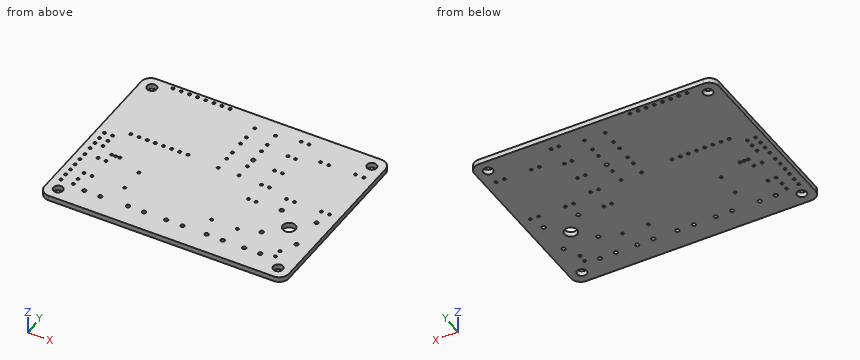
from build123d import *

# Parameters (mm, degrees)
ESQUISSE1_R        = 1.5
ESQUISSE1_R_2      = 0.449122519
ESQUISSE1_R_3      = 0.425258014
ESQUISSE1_R_4      = 0.43212249
ESQUISSE1_R_5      = 0.6
ESQUISSE1_R_6      = 2
BOSS_EXTRU_1_DEPTH = 1.6


with BuildPart() as part:
    # Esquisse1 → Boss.-Extru.1 (new body)
    with BuildSketch(Plane.XY):
        with BuildLine():
            Line((5.620364973, 58.899605158), (75.820364973, 58.899605158))
            ThreePointArc((75.820364973, 58.899605158), (77.941685316, 58.020925502), (78.820364973, 55.899605158))
            Line((78.820364973, 55.899605158), (78.820364973, 3.479605158))
            ThreePointArc((78.820364973, 3.479605158), (77.941685316, 1.358284815), (75.820364973, 0.479605158))
            Line((75.820364973, 0.479605158), (5.620364973, 0.479605158))
            ThreePointArc((5.620364973, 0.479605158), (3.499044629, 1.358284815), (2.620364973, 3.479605158))
            Line((2.620364973, 3.479605158), (2.620364973, 55.899605158))
            ThreePointArc((2.620364973, 55.899605158), (3.499044629, 58.020925502), (5.620364973, 58.899605158))
        make_face()
        with Locations((6.430364973, 55.089605158)):
            Circle(ESQUISSE1_R, mode=Mode.SUBTRACT)
        with Locations((75.010364973, 4.289605158)):
            Circle(ESQUISSE1_R, mode=Mode.SUBTRACT)
        with Locations((6.430364973, 4.289605158)):
            Circle(ESQUISSE1_R, mode=Mode.SUBTRACT)
        with Locations((75.010364973, 55.089605158)):
            Circle(ESQUISSE1_R, mode=Mode.SUBTRACT)
        with Locations((11.552831362, 57.615365404)):
            Circle(ESQUISSE1_R_2, mode=Mode.SUBTRACT)
        with Locations((14.1370916, 57.615365404)):
            Circle(ESQUISSE1_R_3, mode=Mode.SUBTRACT)
        with Locations((16.688639683, 57.615365404)):
            Circle(ESQUISSE1_R_4, mode=Mode.SUBTRACT)
        with Locations((19.199619548, 57.582653249)):
            Circle(ESQUISSE1_R_2, mode=Mode.SUBTRACT)
        with Locations((21.783879785, 57.582653249)):
            Circle(ESQUISSE1_R_3, mode=Mode.SUBTRACT)
        with Locations((24.335427868, 57.582653249)):
            Circle(ESQUISSE1_R_4, mode=Mode.SUBTRACT)
        with Locations((26.821551641, 57.582653249)):
            Circle(ESQUISSE1_R_2, mode=Mode.SUBTRACT)
        with Locations((29.405811879, 57.582653249)):
            Circle(ESQUISSE1_R_3, mode=Mode.SUBTRACT)
        with Locations((11.575035578, 34.708039908)):
            Circle(ESQUISSE1_R_2, mode=Mode.SUBTRACT)
        with Locations((14.159295816, 34.708039908)):
            Circle(ESQUISSE1_R_3, mode=Mode.SUBTRACT)
        with Locations((16.710843899, 34.708039908)):
            Circle(ESQUISSE1_R_4, mode=Mode.SUBTRACT)
        with Locations((19.221823764, 34.675327753)):
            Circle(ESQUISSE1_R_2, mode=Mode.SUBTRACT)
        with Locations((21.806084001, 34.675327753)):
            Circle(ESQUISSE1_R_3, mode=Mode.SUBTRACT)
        with Locations((24.357632084, 34.675327753)):
            Circle(ESQUISSE1_R_4, mode=Mode.SUBTRACT)
        with Locations((26.843755857, 34.675327753)):
            Circle(ESQUISSE1_R_2, mode=Mode.SUBTRACT)
        with Locations((29.428016095, 34.675327753)):
            Circle(ESQUISSE1_R_3, mode=Mode.SUBTRACT)
        with Locations((53.163306818, 54.832264293)):
            Circle(ESQUISSE1_R_3, mode=Mode.SUBTRACT)
        with Locations((55.540433341, 54.832264293)):
            Circle(ESQUISSE1_R_3, mode=Mode.SUBTRACT)
        with Locations((55.570147422, 47.522600237)):
            Circle(ESQUISSE1_R_3, mode=Mode.SUBTRACT)
        with Locations((53.1930209, 47.611742482)):
            Circle(ESQUISSE1_R_3, mode=Mode.SUBTRACT)
        with Locations((53.163306818, 40.420934752)):
            Circle(ESQUISSE1_R_3, mode=Mode.SUBTRACT)
        with Locations((55.570147422, 40.420934752)):
            Circle(ESQUISSE1_R_3, mode=Mode.SUBTRACT)
        with Locations((53.14142812, 33.298983102)):
            Circle(ESQUISSE1_R_3, mode=Mode.SUBTRACT)
        with Locations((55.557053239, 33.3399259)):
            Circle(ESQUISSE1_R_3, mode=Mode.SUBTRACT)
        with Locations((55.557053239, 26.17493614)):
            Circle(ESQUISSE1_R_3, mode=Mode.SUBTRACT)
        with Locations((53.182370918, 26.17493614)):
            Circle(ESQUISSE1_R_3, mode=Mode.SUBTRACT)
        with Locations((62.066958221, 31.292785969)):
            Circle(ESQUISSE1_R_3, mode=Mode.SUBTRACT)
        with Locations((64.646354535, 31.292785969)):
            Circle(ESQUISSE1_R_3, mode=Mode.SUBTRACT)
        with Locations((72.998685456, 31.25184317)):
            Circle(ESQUISSE1_R_3, mode=Mode.SUBTRACT)
        with Locations((75.537138971, 31.292785969)):
            Circle(ESQUISSE1_R_3, mode=Mode.SUBTRACT)
        with Locations((75.57808177, 49.79893095)):
            Circle(ESQUISSE1_R_3, mode=Mode.SUBTRACT)
        with Locations((72.998685456, 49.839873749)):
            Circle(ESQUISSE1_R_3, mode=Mode.SUBTRACT)
        with Locations((64.646354535, 49.757988152)):
            Circle(ESQUISSE1_R_3, mode=Mode.SUBTRACT)
        with Locations((62.10790102, 49.757988152)):
            Circle(ESQUISSE1_R_3, mode=Mode.SUBTRACT)
        with Locations((49.018752461, 13.440847602)):
            Circle(ESQUISSE1_R_3, mode=Mode.SUBTRACT)
        with Locations((57.05002029, 13.440847602)):
            Circle(ESQUISSE1_R_3, mode=Mode.SUBTRACT)
        with Locations((5.102916939, 31.656431458)):
            Circle(ESQUISSE1_R_3, mode=Mode.SUBTRACT)
        with Locations((7.643442377, 31.677780411)):
            Circle(ESQUISSE1_R_3, mode=Mode.SUBTRACT)
        with Locations((7.643442377, 29.115906021)):
            Circle(ESQUISSE1_R_3, mode=Mode.SUBTRACT)
        with Locations((7.622093423, 26.511333724)):
            Circle(ESQUISSE1_R_3, mode=Mode.SUBTRACT)
        with Locations((5.102916939, 26.55403163)):
            Circle(ESQUISSE1_R_3, mode=Mode.SUBTRACT)
        with Locations((5.081567986, 29.073208114)):
            Circle(ESQUISSE1_R_3, mode=Mode.SUBTRACT)
        with Locations((5.081567986, 23.970808287)):
            Circle(ESQUISSE1_R_3, mode=Mode.SUBTRACT)
        with Locations((11.56492709, 24.417750649)):
            Circle(ESQUISSE1_R_3, mode=Mode.SUBTRACT)
        with Locations((12.845140115, 24.358205857)):
            Circle(ESQUISSE1_R_3, mode=Mode.SUBTRACT)
        with Locations((14.12535314, 24.417750649)):
            Circle(ESQUISSE1_R_3, mode=Mode.SUBTRACT)
        with Locations((5.134089571, 20.993925117)):
            Circle(ESQUISSE1_R_3, mode=Mode.SUBTRACT)
        with Locations((5.044772383, 18.433499068)):
            Circle(ESQUISSE1_R_3, mode=Mode.SUBTRACT)
        with Locations((5.044772383, 15.843300623)):
            Circle(ESQUISSE1_R_3, mode=Mode.SUBTRACT)
        with Locations((5.074544779, 13.342419365)):
            Circle(ESQUISSE1_R_3, mode=Mode.SUBTRACT)
        with Locations((5.044772383, 10.781993316)):
            Circle(ESQUISSE1_R_3, mode=Mode.SUBTRACT)
        with Locations((5.074544779, 8.281112058)):
            Circle(ESQUISSE1_R_3, mode=Mode.SUBTRACT)
        with Locations((9.004501041, 13.759232908)):
            Circle(ESQUISSE1_R_3, mode=Mode.SUBTRACT)
        with Locations((9.034273437, 21.380966264)):
            Circle(ESQUISSE1_R_3, mode=Mode.SUBTRACT)
        with Locations((11.594699486, 21.261876681)):
            Circle(ESQUISSE1_R_3, mode=Mode.SUBTRACT)
        with Locations((21.747086496, 21.351193868)):
            Circle(ESQUISSE1_R_3, mode=Mode.SUBTRACT)
        with Locations((21.747086496, 13.759232908)):
            Circle(ESQUISSE1_R_3, mode=Mode.SUBTRACT)
        with Locations((11.535154694, 13.729460512)):
            Circle(ESQUISSE1_R_3, mode=Mode.SUBTRACT)
        with Locations((8.885411457, 10.781993316)):
            Circle(ESQUISSE1_R_3, mode=Mode.SUBTRACT)
        with Locations((8.885411457, 8.281112058)):
            Circle(ESQUISSE1_R_3, mode=Mode.SUBTRACT)
        with Locations((39.348557903, 53.619405616)):
            Circle(ESQUISSE1_R_3, mode=Mode.SUBTRACT)
        with Locations((45.83038937, 53.619405616)):
            Circle(ESQUISSE1_R_3, mode=Mode.SUBTRACT)
        with Locations((45.863629531, 49.09874367)):
            Circle(ESQUISSE1_R_3, mode=Mode.SUBTRACT)
        with Locations((39.348557903, 49.09874367)):
            Circle(ESQUISSE1_R_3, mode=Mode.SUBTRACT)
        with Locations((39.348557903, 45.94092834)):
            Circle(ESQUISSE1_R_3, mode=Mode.SUBTRACT)
        with Locations((45.896869692, 45.907688179)):
            Circle(ESQUISSE1_R_3, mode=Mode.SUBTRACT)
        with Locations((45.863629531, 41.486746717)):
            Circle(ESQUISSE1_R_5, mode=Mode.SUBTRACT)
        with Locations((39.348557903, 41.453506556)):
            Circle(ESQUISSE1_R_3, mode=Mode.SUBTRACT)
        with Locations((45.856335407, 38.34537897)):
            Circle(ESQUISSE1_R_3, mode=Mode.SUBTRACT)
        with Locations((39.350135574, 38.370943606)):
            Circle(ESQUISSE1_R_3, mode=Mode.SUBTRACT)
        with Locations((39.350135574, 33.858785372)):
            Circle(ESQUISSE1_R_3, mode=Mode.SUBTRACT)
        with Locations((45.856335407, 33.8076561)):
            Circle(ESQUISSE1_R_3, mode=Mode.SUBTRACT)
        with Locations((71.852738685, 10.806937061)):
            Circle(ESQUISSE1_R_3, mode=Mode.SUBTRACT)
        with Locations((71.870001894, 8.251982162)):
            Circle(ESQUISSE1_R_3, mode=Mode.SUBTRACT)
        with Locations((12.887042224, 7.217406275)):
            Circle(ESQUISSE1_R_5, mode=Mode.SUBTRACT)
        with Locations((17.87612986, 7.160279318)):
            Circle(ESQUISSE1_R_5, mode=Mode.SUBTRACT)
        with Locations((26.461748825, 7.28752809)):
            Circle(ESQUISSE1_R_5, mode=Mode.SUBTRACT)
        with Locations((31.521661116, 7.222238899)):
            Circle(ESQUISSE1_R_5, mode=Mode.SUBTRACT)
        with Locations((38.409670751, 7.222238899)):
            Circle(ESQUISSE1_R_5, mode=Mode.SUBTRACT)
        with Locations((43.534872233, 7.189594304)):
            Circle(ESQUISSE1_R_5, mode=Mode.SUBTRACT)
        with Locations((51.010484586, 7.254883494)):
            Circle(ESQUISSE1_R_5, mode=Mode.SUBTRACT)
        with Locations((56.070396878, 7.189594304)):
            Circle(ESQUISSE1_R_5, mode=Mode.SUBTRACT)
        with Locations((62.729894345, 7.222238899)):
            Circle(ESQUISSE1_R_5, mode=Mode.SUBTRACT)
        with Locations((67.724517445, 7.222238899)):
            Circle(ESQUISSE1_R_5, mode=Mode.SUBTRACT)
        with Locations((63.404629266, 26.427964058)):
            Circle(ESQUISSE1_R_5, mode=Mode.SUBTRACT)
        with Locations((74.222112873, 26.389874327)):
            Circle(ESQUISSE1_R_5, mode=Mode.SUBTRACT)
        with Locations((74.184023142, 15.610480451)):
            Circle(ESQUISSE1_R_5, mode=Mode.SUBTRACT)
        with Locations((63.404629266, 15.534300989)):
            Circle(ESQUISSE1_R_5, mode=Mode.SUBTRACT)
        with Locations((68.851460801, 20.981132523)):
            Circle(ESQUISSE1_R_6, mode=Mode.SUBTRACT)
    extrude(amount=BOSS_EXTRU_1_DEPTH)


solid = part.part
Check sheet for the modelled part. Datum: model origin and axes. Units: mm. Give positions to 0.01 mm unless a question says otherwise; leave off trailing zeros. One line per item, written item: value. Start each with the question number.
Item 1: Material ranges on probe 1 along X at (y, z) = (4.5, 1.1); probe 2 along X at (y, z) = (55, 0.6); probe 3 along Y at (x, z) = (68, 1.35), recorded low to high. Write a range as from..to.
Item 2: Section check A-A on z = 0.8. State how many separate pieces and enclosed holes the cut face has, then the cut area to 3 significant figures.
Item 3: Gauge pin test, flat end, axial feed: pin 1 (1 mm diameter, centred on x = 24, y = 31.5, fed in from -Z). Record the tip position at first contact, or that the pin passes through.
Results list:
1. probe 1: 2.62..4.95, 7.92..73.53, 76.5..78.82
1. probe 2: 2.62..4.93, 7.93..52.77, 53.55..55.15, 55.93..73.51, 76.51..78.82
1. probe 3: 0.48..6.69, 7.76..19.17, 22.79..58.9
2. separate pieces: 1
2. enclosed holes: 93
2. area: 4,340 mm²
3. pin 1: z = 0
